from build123d import *

# Parameters (mm, degrees)
BOSS_EXTRUDE1_DEPTH = 70
SKETCH2_R           = 25
CUT_EXTRUDE1_DEPTH  = 106.830052443
SKETCH3_OUTSIDE_W   = 237.528
SKETCH3_OUTSIDE_H   = 221.452
SKETCH3_OUTSIDE_R   = 40
CUT_EXTRUDE2_DEPTH  = 70
CUT_EXTRUDE2_DRAFT  = -30
SKETCH6_W           = 12
SKETCH6_H           = 28.841258608
CUT_EXTRUDE3_DEPTH  = 30
CIRPATTERN1_COUNT   = 6


with BuildPart() as part:
    # Sketch1 → Boss-Extrude1 (new body)
    with BuildSketch(Plane.XY):
        Polygon((60, 0), (30, 51.961524227), (-30, 51.961524227), (-60, 0), (-30, -51.961524227), (30, -51.961524227), align=None)
    extrude(amount=BOSS_EXTRUDE1_DEPTH)

    # Sketch2 → Cut-Extrude1 (cut, through all)
    with BuildSketch(Plane.XY.offset(70)):
        Circle(SKETCH2_R)
    extrude(amount=-CUT_EXTRUDE1_DEPTH, mode=Mode.SUBTRACT)


with BuildPart() as cut_extrude2_tool:
    # Sketch3 outside → Cut-Extrude2 (with draft: the straight prism first)
    with BuildSketch(Plane.XY.offset(70)):
        Rectangle(SKETCH3_OUTSIDE_W, SKETCH3_OUTSIDE_H)
        Circle(SKETCH3_OUTSIDE_R, mode=Mode.SUBTRACT)
    extrude(amount=-CUT_EXTRUDE2_DEPTH)
    # Cut-Extrude2: the draft: its side faces are tilted about the plane it starts from
    cut_extrude2_sides = [cut_extrude2_tool.faces().sort_by_distance(p)[0] for p in [
        (0, -110.726, 35),
        (118.764, 0, 35),
        (0, 110.726, 35),
        (-118.764, 0, 35),
        (-40, 0, 35),
    ]]
    draft(cut_extrude2_sides, Plane.XY.offset(70), CUT_EXTRUDE2_DRAFT)


with BuildPart() as part_1:
    add(part.part)

    # Cut-Extrude2: cut by cut_extrude2_tool
    add(cut_extrude2_tool.part, mode=Mode.SUBTRACT)

    # Sketch6 → Cut-Extrude3 (cut)
    with BuildSketch(Plane.XY.offset(70)):
        with Locations((0, -38.689951503)):
            Rectangle(SKETCH6_W, SKETCH6_H)
    cut_extrude3 = extrude(amount=-CUT_EXTRUDE3_DEPTH, mode=Mode.SUBTRACT)

    # CirPattern1: Cut-Extrude3 ×6 about axis
    cirpattern1_axis = Axis((0, 0, 0), (0, 0, 1))
    for i in range(1, CIRPATTERN1_COUNT):
        add(cut_extrude3.rotate(cirpattern1_axis, i * 360 / CIRPATTERN1_COUNT), mode=Mode.SUBTRACT)


solid = part_1.part
Source: CAD feature listing. Evaluate the final solid. Frame: model axes, mm. A direction names the side the tool comes from. Give positions to 0.01 mm unless a question says otherwise; leave off trailing zeros. Order: outer loops, then holes, each group sorted by start corner. A loop starts at its lowest first (then second) coordinate and runs counter-clockwise, first axis right, second up. Notation, with made-up numbers: (-3.5, 23) -> (0.5, 23) arc R34 cw to (0.5, 59) -> close; hole circle Ø7 at (8, 78.25). An arc over 180 degrees is marked (long way). Write item = value, one per line.
Q1. Pull-direction query (Y, two-part tool) for faces 4 (the face through (-33, -19, 40)), 5 (the face through (-23.582, 41.391, 56.771)), 6 (the face through (16, 29, 70)); classes: released by +Y, released by -Y, zero draft, split by the parting line, or undercut.
Data:
face_4 = undercut
face_5 = released by +Y
face_6 = zero draft
Q2. Cut plane B-B, the plane x = 0. Output: boundary loops of the cut face in (y, z).
Data:
outline = (-51.96, 0) -> (-25, 0) -> (-25, 40) -> (-51.96, 40) -> close; (25, 0) -> (51.96, 0) -> (51.96, 40) -> (25, 40) -> close
Q3. Pin query (flat end, axial travel): pin 1 (6 mm diameter, centred on x = -1.5, y = 44, fed in from +Z); pin 2 (12 mm diameter, centred on x = -31.5, z = 49, fed in from +Y); pin 3 (6 mm diameter, centred on y = -21, z = 18, fed in from -X). Return the tip coordinate at first contact, or that it passes through.
Data:
pin_1 = 40
pin_2 = 47.29
pin_3 = -49.61
Q4. Material intervals for line 1 (X direction, y = 0, z = 23); line 2 (Y direction, x = 0, z = 33); line 3 (Z direction, x = 29, y = 12), sorted ascending. Write a range as from..to.
Data:
line_1 = -60..-25, 25..60
line_2 = -51.96..-25, 25..51.96
line_3 = 0..40
Q5. Set-up query: faces 1 (the face through (0, -38, 40)), 2 (the face through (-27.51, 22.81, 55.21)), 3 (the face through (0, -51.962, 24)). Return all of +Z, -Z, +X, -X, +Y, -Y with unobstructed straight access to the full face (end or side cutting, diameter ignored); none if empty.
Data:
face_1 = +Z, +Y, -Y
face_2 = +Z
face_3 = +Z, -Z, +X, -X, -Y
Q6. Cut plane A-A, the plane z = 20. Output: boundary loops of the cut face in (x, y).
Data:
outline = (-60, 0) -> (-30, -51.96) -> (30, -51.96) -> (60, 0) -> (30, 51.96) -> (-30, 51.96) -> close; hole circle Ø50 at (0, 0)
Q7. Cut plane C-C, the plane z = 55. Output: boundary loops of the cut face in (x, y).
Data:
outline = (-44.82, -18.95) -> (-24.02, -6.94) arc R25 cw to (-24.02, 6.94) -> (-44.82, 18.95) arc R48.66 ccw to start; (-38.82, -29.34) arc R48.66 ccw to (-6, -48.29) -> (-6, -24.27) arc R25 cw to (-18.02, -17.33) -> close; (-38.82, 29.34) -> (-18.02, 17.33) arc R25 cw to (-6, 24.27) -> (-6, 48.29) arc R48.66 ccw to start; (6, -48.29) arc R48.66 ccw to (38.82, -29.34) -> (18.02, -17.33) arc R25 cw to (6, -24.27) -> close; (6, 24.27) arc R25 cw to (18.02, 17.33) -> (38.82, 29.34) arc R48.66 ccw to (6, 48.29) -> close; (24.02, -6.94) -> (44.82, -18.95) arc R48.66 ccw to (44.82, 18.95) -> (24.02, 6.94) arc R25 cw to start
Q8. Cut plane D-D, the plane z = 46.5. State how many separate pieces and enclosed holes the cut face has, and give its area (3 significant figures).
Data:
separate_pieces = 6
enclosed_holes = 0
area = 4,920 mm^2
